Can you work these out from the model? Positions are in its coordinate system, mm. Face numbers are marked on the shaded views. A direction names the side the tool comes from. Give positions to 0.01 mm unless a question says otherwise; leave off trailing zeros. Loops run counter-clockwise (first coordinate to the right, second up) from the corner with the lowest first, then second, coordinate; pieces in that order, holes last. Notation, with made-up numbers: M -9.5,87.25 L -5.5,87.25 A19 ccw -5.5,97.25 Z; hole C 12,83.25 d2. An arc over 180 degrees is marked long. Use CSV: the item, a comma, the result in double quotes.
from build123d import *

# Parameters (mm, degrees)
BOSS_EXTRUDE1_DEPTH      = 1
BOSS_EXTRUDE2_DEPTH      = 18
BOSS_EXTRUDE2_DEPTH_BACK = 18.972201
SKETCH3_R                = 59.910539196270584
CUT_EXTRUDE1_DEPTH       = 28.593195008632154
CUT_EXTRUDE2_DEPTH       = 28.59319484059837
CUT_EXTRUDE2_DEPTH_BACK  = 28.59319484059837
SKETCH5_R                = 1.4
SKETCH5_R_2              = 1.3999999999999992
SKETCH5_R_3              = 1.400000000000003
SKETCH5_R_4              = 1.3999999999999988
SKETCH5_R_5              = 1.399999999999999
BOSS_EXTRUDE3_DEPTH      = 8.8
CUT_EXTRUDE3_DEPTH       = 28.290738383400775
FILLET1_R                = 2
FILLET2_R                = 0.5


with BuildPart() as part:
    # Sketch1 → Boss-Extrude1 (new body)
    with BuildSketch(Plane(origin=(0, 0, 0), x_dir=(1, 0, 0), z_dir=(0, 1, 0))):
        with BuildLine():
            Line((-1.0000000000000024, 17.97220075561143), (-1.0000000000000024, 18.97220075561143))
            Line((-1.0000000000000024, 18.97220075561143), (0.9999999999999977, 18.97220075561143))
            Line((0.9999999999999977, 18.97220075561143), (0.9999999999999981, 17.97220075561143))
            ThreePointArc((0.9999999999999981, 17.97220075561143), (-3.31e-15, -18), (-1.0000000000000024, 17.97220075561143))
        make_face()
    extrude(amount=BOSS_EXTRUDE1_DEPTH)

    # Sketch2 → Boss-Extrude2 (add, two sides: drawn at the far end of the back side and taken through both)
    with BuildSketch(Plane.XY.offset(-BOSS_EXTRUDE2_DEPTH_BACK)):
        Polygon((-16.1, 8.799999999999999), (-8.100000000000005, 8.799999999999999), (-8.099999999999996, 1), (-16.099999999999998, 1), align=None)
        Polygon((8.099999999999994, 8.799999999999999), (16.099999999999994, 8.799999999999999), (16.100000000000005, 1), (8.100000000000003, 0.9999999999999991), align=None)
    extrude(amount=BOSS_EXTRUDE2_DEPTH + BOSS_EXTRUDE2_DEPTH_BACK)

    # Sketch3 → Cut-Extrude1 (cut, through all)
    with BuildSketch(Plane.XZ):
        Circle(SKETCH3_R)
        with BuildLine():
            Line((-1.000000000000015, -17.97220075561143), (-1.0000000000000024, -18.97220075561143))
            Line((-1.0000000000000024, -18.97220075561143), (0.9999999999999977, -18.97220075561143))
            Line((0.9999999999999977, -18.97220075561143), (0.9999999999999927, -17.972200755611432))
            ThreePointArc((0.9999999999999927, -17.972200755611432), (1.309e-14, 18.000000000000004), (-1.000000000000015, -17.97220075561143))
        make_face(mode=Mode.SUBTRACT)
    extrude(amount=-CUT_EXTRUDE1_DEPTH, mode=Mode.SUBTRACT)

    # Sketch5 → Cut-Extrude2 (cut, two sides: drawn at the far end of the back side and taken through both)
    with BuildSketch(Plane(origin=(0, 0, 0), x_dir=(1, 0, 0), z_dir=(0, 1, 0)).offset(-CUT_EXTRUDE2_DEPTH_BACK)):
        with Locations(Location((0, 0, 0), (0, 0, 180))):
            Circle(SKETCH5_R)
        with Locations(Location((11, -4, 0), (0, 0, 180))):
            Circle(SKETCH5_R_2)
        with Locations(Location((-11, -4, 0), (0, 0, 180))):
            Circle(SKETCH5_R_2)
        with Locations(Location((-11.69134295108996, 6.749999999999895, 0), (0, 0, 180))):
            Circle(SKETCH5_R_3)
        with Locations(Location((1.197e-13, -13.499999999999998, 0), (0, 0, 180))):
            Circle(SKETCH5_R_4)
        with Locations(Location((11.691342951089881, 6.750000000000103, 0), (0, 0, 180))):
            Circle(SKETCH5_R_5)
    extrude(amount=CUT_EXTRUDE2_DEPTH + CUT_EXTRUDE2_DEPTH_BACK, mode=Mode.SUBTRACT)

    # Sketch6 → Boss-Extrude3 (add)
    with BuildSketch(Plane.XZ):
        with BuildLine():
            Line((-8.097530487747482, -15.075758146973973), (8.097530487747482, -15.075758146973973))
            Line((8.097530487747482, -15.075758146973973), (8.09753048774748, -16.075758146973975))
            ThreePointArc((8.09753048774748, -16.075758146973975), (4.646545909149893, -17.38992843901787), (0.9999999999999927, -17.972200755611432))
            Line((0.9999999999999927, -17.972200755611432), (0.9999999999999977, -18.97220075561143))
            Line((0.9999999999999977, -18.97220075561143), (-1.0000000000000024, -18.97220075561143))
            Line((-1.0000000000000024, -18.97220075561143), (-1.000000000000015, -17.97220075561143))
            ThreePointArc((-1.000000000000015, -17.97220075561143), (-4.646545909149902, -17.38992843901787), (-8.097530487747482, -16.075758146973975))
            Line((-8.097530487747482, -16.075758146973975), (-8.097530487747482, -15.075758146973973))
        make_face()
    extrude(amount=-BOSS_EXTRUDE3_DEPTH)

    # Sketch7 → Cut-Extrude3 (cut, through all)
    with BuildSketch(Plane(origin=(0, 1, 0), x_dir=(1, 0, 0), z_dir=(0, 1, 0))):
        with BuildLine():
            Line((16.099999999999994, 8.049223565040313), (16.099999999999994, -8.049223565040313))
            ThreePointArc((16.099999999999994, -8.049223565040313), (18.000000000000004, 0), (16.099999999999994, 8.049223565040313))
        make_face()
        with BuildLine():
            Line((-16.099999999999998, -8.049223565040306), (-16.099999999999998, 8.049223565040306))
            ThreePointArc((-16.099999999999998, 8.049223565040306), (-18.000000000000004, 2.2e-15), (-16.099999999999998, -8.049223565040306))
        make_face()
    extrude(amount=-CUT_EXTRUDE3_DEPTH, mode=Mode.SUBTRACT)

    # Fillet1
    # the kernel refuses this fillet: 2 mm, written as the material it takes off along each edge
    with BuildSketch(Plane(origin=(-3.872e-14, 0, -5.4e-16), x_dir=(0.9828239646934485, 0, 0.1845455348260998), z_dir=(0.1845455348260998, 0, -0.9828239646934485))) as fillet1_piece_1:
        with BuildLine():
            CenterArc((17.999999999999872 - FILLET1_R, -FILLET1_R), FILLET1_R, 6.36e-15, 90)
            Line((17.999999999999872, -FILLET1_R), (17.999999999999872, 0))
            Line((17.999999999999872, 0), (17.999999999999872 - FILLET1_R, 0))
        make_face()
    revolve(axis=Axis((-3.872e-14, 0, -5.4e-16), (0, -1, 0)), revolution_arc=158.7307255035683, mode=Mode.SUBTRACT)
    with BuildSketch(Plane(origin=(-3.872e-14, 0, -5.4e-16), x_dir=(0.4498628048748618, 0, -0.8930976748318865), z_dir=(-0.8930976748318865, 0, -0.4498628048748618))) as fillet1_piece_2:
        with BuildLine():
            CenterArc((18.000000000000004 - FILLET1_R, -FILLET1_R), FILLET1_R, 6.36e-15, 90)
            Line((18.000000000000007, -FILLET1_R), (18.000000000000004, 0))
            Line((18.000000000000004, 0), (18.000000000000004 - FILLET1_R, 0))
        make_face()
    revolve(axis=Axis((-3.872e-14, 0, -5.4e-16), (0, -1, 0)), revolution_arc=52.61883467829079, mode=Mode.SUBTRACT)
    with BuildSketch(Plane(origin=(16.099999999999994, 0, 13.049223565040313), x_dir=(-1, 0, 0), z_dir=(0, 0, -1))) as fillet1_piece_3:
        with BuildLine():
            CenterArc((FILLET1_R, FILLET1_R), FILLET1_R, 180, 90)
            Line((0, FILLET1_R), (0, 0))
            Line((0, 0), (FILLET1_R, 0))
        make_face()
    extrude(amount=26.098447130080626, mode=Mode.SUBTRACT)
    with BuildSketch(Plane(origin=(-16.099999999999998, 0, -13.049223565040311), x_dir=(1, 0, 0), z_dir=(0, 0, 1))) as fillet1_piece_4:
        with BuildLine():
            CenterArc((FILLET1_R, FILLET1_R), FILLET1_R, 180, 90)
            Line((0, FILLET1_R), (0, 0))
            Line((0, 0), (FILLET1_R, 0))
        make_face()
    extrude(amount=26.098447130080615, mode=Mode.SUBTRACT)
    with BuildSketch(Plane(origin=(-3.872e-14, 0, -5.4e-16), x_dir=(-0.9827864332200049, 0, -0.18474530218303542), z_dir=(-0.18474530218303542, 0, 0.9827864332200049))) as fillet1_piece_5:
        with BuildLine():
            CenterArc((18.000000000000007 - FILLET1_R, -FILLET1_R), FILLET1_R, 0, 90)
            Line((18.000000000000007 - FILLET1_R, 2.2e-16), (18.000000000000007, 0))
            Line((18.000000000000007, 0), (18.000000000000007, -FILLET1_R))
        make_face()
    revolve(axis=Axis((-3.872e-14, 0, -5.4e-16), (0, -1, 0)), revolution_arc=52.61883467829094, mode=Mode.SUBTRACT)
    with BuildSketch(Plane(origin=(-3.872e-14, 0, -5.4e-16), x_dir=(-0.44986280487485913, 0, -0.8930976748318878), z_dir=(-0.8930976748318878, 0, 0.44986280487485913))) as fillet1_piece_6_section:
        with BuildLine():
            CenterArc((18 - FILLET1_R, -FILLET1_R), FILLET1_R, 0, 89.9999999999999)
            Line((18 - FILLET1_R, 2.2e-16), (18, 0))
            Line((18, 0), (18, -FILLET1_R))
        make_face()
    fillet1_piece_6 = revolve(axis=Axis((-3.872e-14, 0, -5.4e-16), (0, -1, 0)), revolution_arc=39.46607540970417, mode=Mode.PRIVATE)
    fillet1_piece_6 = split(fillet1_piece_6, bisect_by=Plane(origin=(-1.0000000000000024, 0.45992141450225776, -16.842636156243355), z_dir=(-1, 0, 0)), keep=Keep.TOP, mode=Mode.PRIVATE)
    add(fillet1_piece_6, mode=Mode.SUBTRACT)
    with BuildSketch(Plane(origin=(-3.872e-14, 0, -5.4e-16), x_dir=(-0.44986280487485913, 0, -0.8930976748318878), z_dir=(-0.8930976748318878, 0, 0.44986280487485913))) as fillet1_piece_7_section:
        with BuildLine():
            CenterArc((18 - FILLET1_R, -FILLET1_R), FILLET1_R, 0, 89.9999999999999)
            Line((18 - FILLET1_R, 2.2e-16), (18, 0))
            Line((18, 0), (18, -FILLET1_R))
        make_face()
    fillet1_piece_7 = revolve(axis=Axis((-3.872e-14, 0, -5.4e-16), (0, -1, 0)), revolution_arc=39.46607540970417, mode=Mode.PRIVATE)
    fillet1_piece_7 = split(fillet1_piece_7, bisect_by=Plane(origin=(0.9999999999999897, 0.4612121351403519, -17.37087292856804), z_dir=(1, 0, 5e-15)), keep=Keep.TOP, mode=Mode.PRIVATE)
    add(fillet1_piece_7, mode=Mode.SUBTRACT)
    with BuildSketch(Plane(origin=(-3.872e-14, 0, -5.4e-16), x_dir=(-0.22037727986092012, 0, -0.9754147089936167), z_dir=(-0.9754147089936167, 0, 0.22037727986092012))) as fillet1_piece_8_section:
        with BuildLine():
            CenterArc((18.000000000000014 - FILLET1_R, -FILLET1_R), FILLET1_R, 1.272e-14, 90)
            Line((18.000000000000014, -FILLET1_R), (18.000000000000014, 0))
            Line((18.000000000000014, 0), (18.000000000000014 - FILLET1_R, 0))
        make_face()
    fillet1_piece_8 = revolve(axis=Axis((-3.872e-14, 0, -5.4e-16), (0, -1, 0)), revolution_arc=39.46607540970416, mode=Mode.PRIVATE)
    fillet1_piece_8 = split(fillet1_piece_8, bisect_by=Plane(origin=(-1.0000000000000024, 0.4612120759147971, -17.37087269742329), z_dir=(-1, 0, 0)), keep=Keep.TOP, mode=Mode.PRIVATE)
    add(fillet1_piece_8, mode=Mode.SUBTRACT)
    with BuildSketch(Plane(origin=(-3.872e-14, 0, -5.4e-16), x_dir=(-0.22037727986092012, 0, -0.9754147089936167), z_dir=(-0.9754147089936167, 0, 0.22037727986092012))) as fillet1_piece_9_section:
        with BuildLine():
            CenterArc((18.000000000000014 - FILLET1_R, -FILLET1_R), FILLET1_R, 1.272e-14, 90)
            Line((18.000000000000014, -FILLET1_R), (18.000000000000014, 0))
            Line((18.000000000000014, 0), (18.000000000000014 - FILLET1_R, 0))
        make_face()
    fillet1_piece_9 = revolve(axis=Axis((-3.872e-14, 0, -5.4e-16), (0, -1, 0)), revolution_arc=39.46607540970416, mode=Mode.PRIVATE)
    fillet1_piece_9 = split(fillet1_piece_9, bisect_by=Plane(origin=(0.999999999999987, 0.4599214469726478, -16.84263631620444), z_dir=(1, 0, 5e-15)), keep=Keep.TOP, mode=Mode.PRIVATE)
    add(fillet1_piece_9, mode=Mode.SUBTRACT)

    # Fillet2
    fillet2_edges = [part.edges().sort_by_distance(p)[0] for p in [
        (4.646545909149891, 8.8, -17.38992843901787),
        (-4.646545909149905, 8.8, -17.389928439017865),
        (16.099999999999994, 8.799999999999999, 0),
        (-16.1, 8.799999999999999, 0),
        (-12.747992845911156, 8.799999999999999, 12.70781957696123),
        (-12.747992845911165, 8.799999999999999, -12.707819576961219),
        (12.747992845911162, 8.799999999999999, 12.707819576961153),
        (12.74799284591116, 8.799999999999999, -12.707819576961155),
    ]]
    fillet(fillet2_edges, radius=FILLET2_R)


solid = part.part
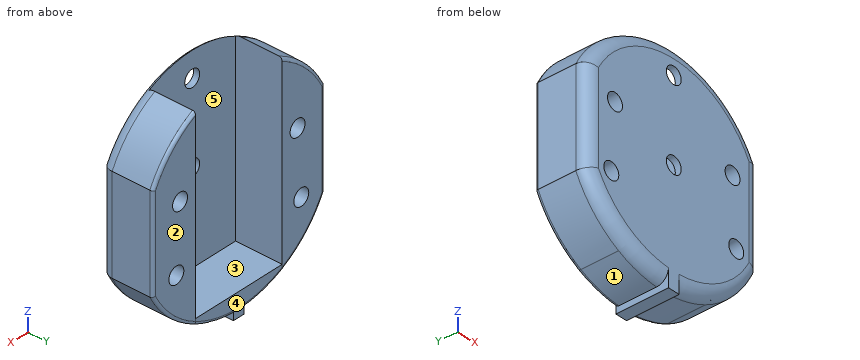
Q1. I want a section at D-D, the plane x = -11. State how many separate pieces and enclosed holes the cut face has, then the cut area to 3 significant figures.
Model answer:
separate pieces,"3"
enclosed holes,"0"
area,"202 mm2"
Q2. I want a section at A-A, the plane z = 0. Please give me the cut outline in (x, y), then the cut area to 3 significant figures.
Model answer:
outline,"M -16.1,2 A2 ccw -14.1,0 L -1.4,0 L -1.4,1 L -8.1,1 L -8.1,8.8 L -15.6,8.8 A0.5 ccw -16.1,8.3 Z; M 1.4,0 L 14.1,0 A2 ccw 16.1,2 L 16.1,8.3 A0.5 ccw 15.6,8.8 L 8.1,8.8 L 8.1,1 L 1.4,1 Z"
area,"152 mm2"
Q3. I want a section at B-B, the plane y = 6.25. Please give me the cut outline in (x, z).
Model answer:
outline,"M -16.1,-8.05 A18 ccw -8.1,-16.07 L -8.1,16.07 A18 ccw -16.1,8.05 Z; M -8.1,-16.08 A18 ccw -1,-17.97 L -1,-18.97 L 1,-18.97 L 1,-17.97 A18 ccw 8.1,-16.08 L 8.1,-15.08 L -8.1,-15.08 Z; M 8.1,-16.07 A18 ccw 16.1,-8.05 L 16.1,8.05 A18 ccw 8.1,16.07 Z; hole C -11.69,-6.75 d2.8; hole C -11,4 d2.8; hole C 11,4 d2.8; hole C 11.69,-6.75 d2.8"
Q4. If we mould it in two halves opening along X, with no side actions, what happens to the marked faces 1, 2 and 3? For each: released by +X, released by -X, zero draft, split by the parting line, or undercut.
Model answer:
face 1,"released by -X"
face 2,"zero draft"
face 3,"undercut"
Q5. I'm going to push flat-ended pins straight in: P1, Ø5, axis at x = 6.5, y = 4.5, coming from the +Z side; P2, Ø1.5, axis at y = 3.5, z = -11, coming from the -X side; P3, Ø1.5, axis at y = 5.5, z = -17, coming from the +X side. Where does each tip first touch, or does it pass through?
Model answer:
P1,"z = 16.07"
P2,"x = -14.8"
P3,"x = 7.74"
Q6. For the marked faces 4 and 5, which set-ups out of +Z, -Z, +X, -X, +Y, -Y let a thin tool reach every point of the face, with its end or its side?
Model answer:
face 4,"+Z, -Z, +X, -X, +Y"
face 5,"+Z, +Y"
Q7. Please list where these lines run through material, in increasing order: L1, parallel to X at y = 2.5, z = 4; L2, parallel to X at y = 2.25, z = 1.5; L3, parallel to Z at x = 11, y = 4. Write a range as from..to.
Model answer:
L1,"-16.1..-12.4, -9.6..-8.1, 8.1..9.6, 12.4..16.1"
L2,"-16.1..-8.1, 8.1..16.1"
L3,"-14.25..-7.97, -5.53..2.6, 5.4..14.25"
Q8. I want a section at C-C, the plane z = -6.75. Please give me the cut outline in (x, y), then the cut area to 3 significant figures.
Model answer:
outline,"M -16.1,2 A2 ccw -14.1,0 L -13.09,0 L -13.09,8.8 L -15.6,8.8 A0.5 ccw -16.1,8.3 Z; M -10.29,0 L 10.29,0 L 10.29,8.8 L 8.1,8.8 L 8.1,1 L -8.1,1 L -8.1,8.8 L -10.29,8.8 Z; M 13.09,0 L 14.1,0 A2 ccw 16.1,2 L 16.1,8.3 A0.5 ccw 15.6,8.8 L 13.09,8.8 Z"
area,"106 mm2"
